Solid Edge part; units mm, degrees
sketch "Sketch1" plane through (0, 0, 0) normal (0, -1, 0) x (1, 0, 0)
  line L0 (21.534, 3.72) -> (57.874, 3.72)
  line L1 (57.874, 3.72) -> (57.874, 2.6)
  line L2 (57.874, 2.6) -> (64.224, 2.6)
  line L3 (64.224, 0) -> (64.224, 2.6)
  line L4 (0, 0) -> (64.224, 0)
  line L5 (0, 0) -> (-45.156, 0)
  line L6 (-45.156, 0) -> (-45.156, 3.26)
  line L7 (-45.156, 3.26) -> (20.744, 3.26)
  line L8 (20.744, 3.26) -> (21.534, 3.72)
revolve "RevolvedProtrusion1" add sketch "Sketch1" angle 360 about axis through (0, 0, 0) along (1, 0, 0)
sketch "Sketch2" plane through (0, 0, 0) normal (0, -1, 0) x (1, 0, 0)
  line L0 (62.924, 1.995) -> (54.704, 1.995)
  line L1 (54.704, 1.995) -> (54.524, 1.695)
  line L2 (54.524, 1.695) -> (51.534, 1.695)
  line L3 (51.534, 1.695) -> (50.514, 0)
  line L4 (50.514, 0) -> (64.224, 0)
  line L5 (64.224, 0) -> (64.224, 2.045)
  line L6 (64.224, 2.045) -> (62.954, 2.045)
  line L7 (62.954, 2.045) -> (62.924, 1.995)
revolve "RevolvedCutout1" cut sketch "Sketch2" angle 360 about axis through (21.534, 0, 0) along (1, 0, 0)
Build history of the part. All positions in model axes, mm. A direction names the side the tool comes from. Coordinates: 2 decimals unless noted, no trailing zeros. Order: outer loops, then holes, each group sorted by start corner. A loop starts at its lowest first (then second) coordinate and runs counter-clockwise, first axis right, second up. Notation, with made-up numbers: (-35, 75) -> (3, 75) arc R21 cw to (3, 102) -> close; hole circle Ø5 at (14.5, -29.5). An arc over 180 degrees is marked (long way). One line per item, written item: value.
(1) Probe line 1 (Y direction, x = 60, z = 0) (3 decimals); line 2 (Z direction, x = 53.7, y = 0) (3 decimals); line 3 (X direction, y = -0.75, z = -2.75). List the from-to ranges inside material, lowest first. Write a range as [from, to].
Checked values:
line 1: [-2.6, -1.995], [1.995, 2.6]
line 2: [-3.72, -1.695], [1.695, 3.72]
line 3: [-45.16, 57.87]
(2) Tool access for faces 4 (the cylindrical face through (61.093, -2.578, -0.338)), 5 (the flat face through (-45.156, 0, 0)), 6 (the cylindrical face through (-11.74, -2.75, 1.75)): list every direction of +Z, -Z, +X, -X, +Y, -Y with a clear straight run to the whole face (end or side of a thin tool).
Checked values:
face 4: +X
face 5: +Z, -Z, -X, +Y, -Y
face 6: -X
(3) Mould opens along Z. For faces 1 (the cylindrical face through (39.958, -0.164, -3.716)), 2 (the flat face through (64.224, 1, -2)), 3 (the cylindrical face through (58.756, -1.214, -1.583)) say: pulls with the +Z half, pulls with the -Z half, needs draft (parallel to the pull), parting line crosses it, or undercut.
Checked values:
face 1: parting line crosses it
face 2: needs draft
face 3: undercut
(4) Slice it at A-A, the plane x = 38.5. List the corners of the cut face in (y, z), plus the area to 3 significant figures.
Checked values:
outline: circle Ø7.44 at (0, 0)
area: 43.5 mm2
(5) Drop flat-ended pins along their axis: pin 1 Ø3.5 at (y, z) = (0, 0) entering from +X; pin 2 Ø3 at (x, z) = (-8, 1) entering from +Y; pin 3 Ø2 at (x, y) = (38.5, -2) entering from +Z; pin 4 Ø1 at (y, z) = (0, 3) entering from +X. Give the stop position or say it passes through.
Checked values:
pin 1: x = 54.56
pin 2: y = 3.26
pin 3: z = 3.58
pin 4: x = 64.22
(6) Slice it at B-B, the plane x = 10.5. List the corners of the cut face in (y, z).
Checked values:
outline: circle Ø6.52 at (0, 0)
